Design review of the part shown in the three views and the two pictorial views. Dimensions are in mm from the part's minimum x, y and z. Round coordinates to 2 decimals unless told otherwise and drop trailing zeros. Write each loop counter-clockwise with the first axis right and the second up, starting at its lowest first coordinate (ties: lowest second). Pieces come first, ordered by that corner, then holes. Notation, with made-up numbers: (-38.75, 71.5) -> (-29.75, 71.5) arc R13 ccw to (-29.75, 75.5) -> close; hole circle Ø9 at (73, 50.5). An arc over 180 degrees is marked (long way). Answer as a JSON object with one key per item and string values. Group by question number.
1) We need section B-B, the plane z = 15. Write out the cut boundary in (x, y).
2) We need section D-D, the plane y = 7.75. Write out the cut boundary in (x, z), then the cut area to 3 significant figures.
3) Mouldability with a two-part tool opening along Y and no side actions: class the marked faces 1, 2 and 3 as pulls with the +Y half, pulls with the -Y half, needs draft (parallel to the pull), parting line crosses it, or undercut.
4) To check wall thickness, follow probe 1 along Y at (x, z) = (1.45, 26); probe 2 along Y at (x, z) = (1.05, 15); probe 3 along Z at (x, y) = (2, 16.25). State the ranges of each line that lie inside material, in increasing order. Write a range as [from, to].
5) Insertion check: pin 1 Ø5 at (y, z) = (6, 15) entering from -X. The pin has a flat end and moves straight along its axis. Give the tip position at first contact, or say it passes through.
6) We need section C-C, the plane z = 26. Write out the cut boundary in (x, y), then the cut area to 3 significant figures.
7) We need section A-A, the plane y = 16. Write out the cut boundary in (x, z).
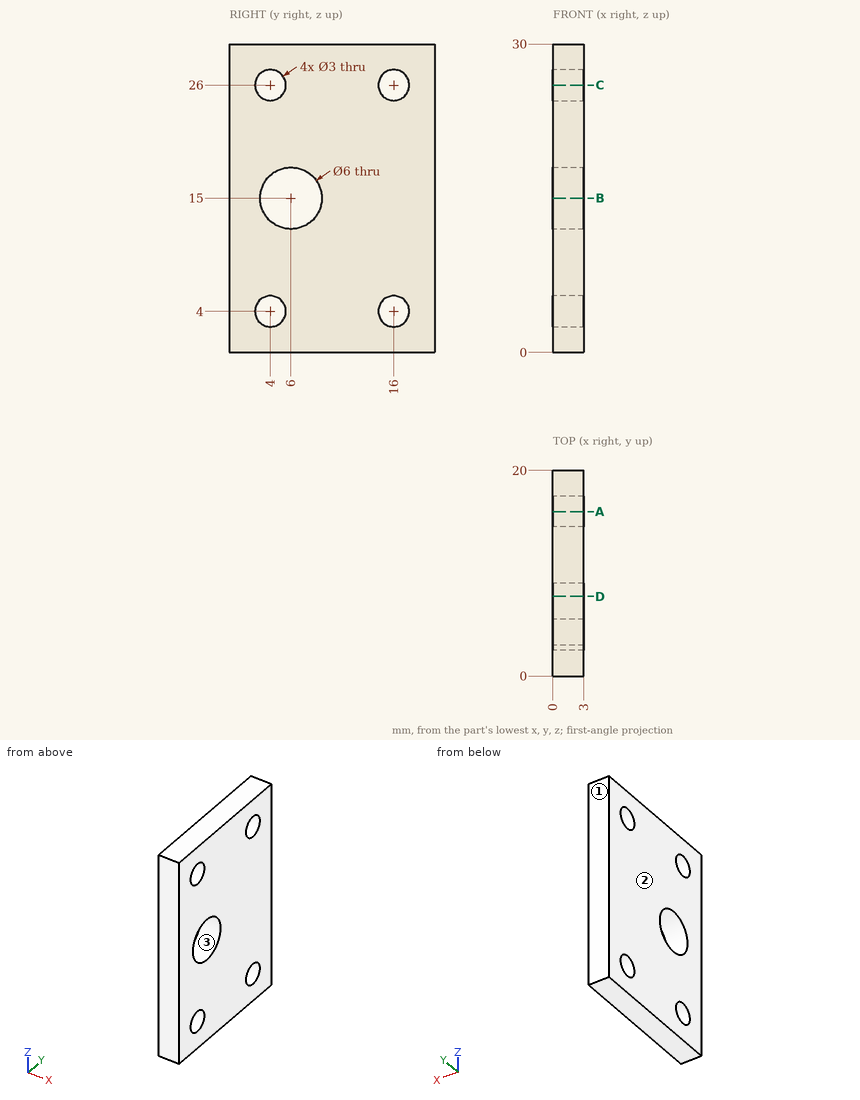
Here are the results:
{
 "1": {"outline": "(0, 0) -> (3, 0) -> (3, 3) -> (0, 3) -> close; (0, 9) -> (3, 9) -> (3, 20) -> (0, 20) -> close"},
 "2": {"outline": "(0, 0) -> (3, 0) -> (3, 12.56) -> (0, 12.56) -> close; (0, 17.44) -> (3, 17.44) -> (3, 30) -> (0, 30) -> close", "area": "75.4 mm^2"},
 "3": {"face 1": "pulls with the +Y half", "face 2": "needs draft", "face 3": "undercut"},
 "4": {"probe 1": "y = [0, 2.5], [5.5, 14.5], [17.5, 20]", "probe 2": "y = [0, 3], [9, 20]", "probe 3": "z = [0, 2.52], [5.48, 24.52], [27.48, 30]"},
 "5": {"pin 1": "passes through"},
 "6": {"outline": "(0, 0) -> (3, 0) -> (3, 2.5) -> (0, 2.5) -> close; (0, 5.5) -> (3, 5.5) -> (3, 14.5) -> (0, 14.5) -> close; (0, 17.5) -> (3, 17.5) -> (3, 20) -> (0, 20) -> close", "area": "42.0 mm^2"},
 "7": {"outline": "(0, 0) -> (3, 0) -> (3, 2.5) -> (0, 2.5) -> close; (0, 5.5) -> (3, 5.5) -> (3, 24.5) -> (0, 24.5) -> close; (0, 27.5) -> (3, 27.5) -> (3, 30) -> (0, 30) -> close"}
}
